Here's how the part is built. I have some questions about the finished solid (model axes, mm). Coordinates: 2 decimals unless noted, no trailing zeros. Loops run counter-clockwise (first coordinate to the right, second up) from the corner with the lowest first, then second, coordinate; pieces in that order, holes last. Notation, with made-up numbers: (31, 35.25) -> (67, 35.25) arc R32 cw to (67, 66.25) -> close; hole circle Ø7 at (-18.75, -4.5). An arc over 180 degrees is marked (long way). Answer as a JSON object with one key per item and string values. Group by question number.
Q1. I'm going to push flat-ended pins straight in: pin 1 (5 mm diameter, centred on x = -3.5, z = -1.5, fed in from -Y); pin 2 (5 mm diameter, centred on x = -7, z = -7.5, fed in from -Y). Where does each tip first touch, or does it pass through?
Q2. I want a section at C-C on z = 0.25. Write out the boundary of the cut face in (x, y), then the cut area to 3 significant figures.
Q3. I need wall thicknesses on line 1 (Z direction, x = -0.75, y = 0.05); line 2 (Z direction, x = 1.25, y = 0.8); line 3 (X direction, y = 0.25, z = -2). Which ranges of each line are inside material? Lowest first, please.
Q4. I want a section at A-A on y = 0. Write out the boundary of the cut face in (x, z), then the cut area to 3 significant figures.
Q5. I want a section at B-B on x = 4.5. Write out the boundary of the cut face in (y, z).
Autodesk Inventor part; units mm, degrees
ref_plane "YZ Plane" through (0, 0, 0) normal (1, 0, 0) x (0, 1, 0)
ref_plane "XZ Plane" through (0, 0, 0) normal (0, 1, 0) x (-1, 0, 0)
ref_plane "XY Plane" through (0, 0, 0) normal (0, 0, 1) x (1, 0, 0)
sketch "Эскиз1" plane through (0, 0, 0) normal (0, 1, 0) x (-1, 0, 0)
  line L0 (4.3898, 6.6229) -> (-5.6102, 6.6229)
  line L1 (-9.6102, 2.6229) -> (-9.6102, -7.3771)
  line L2 (-5.6102, -11.3771) -> (4.3898, -11.3771)
  line L3 (8.3898, -7.3771) -> (8.3898, 2.6229)
  arc A0 (8.3898, 2.6229) -> (4.3898, 6.6229) centre (4.3898, 2.6229) ccw
  arc A1 (4.3898, -11.3771) -> (8.3898, -7.3771) centre (4.3898, -7.3771) ccw
  arc A2 (-9.6102, -7.3771) -> (-5.6102, -11.3771) centre (-5.6102, -7.3771) ccw
  arc A3 (-5.6102, 6.6229) -> (-9.6102, 2.6229) centre (-5.6102, 2.6229) ccw
  point P0 (0, 0)
  point P1 (-9.6102, -11.3771)
  point P2 (-9.6102, 6.6229)
  point P3 (8.3898, -11.3771)
  point P4 (0, -11.3771)
  dimension "d0" = 18
  dimension "d1" = 18
  dimension "d2" = 4
sketch "Эскиз2" plane through (0, 0, 0) normal (0, 1, 0) x (-1, 0, 0)
  point P0 (0, 0)
ref_plane "РабПлоскость1" through (0, 0, -11.3771) normal (-1, 0, 0) x (0, -1, 0)
sketch "Эскиз3" plane through (0, 0, -11.3771) normal (-1, 0, 0) x (0, -1, 0)
  circle A0 centre (0, 0) radius 1.0246
  point P0 (0, 11.3771)
sweep "Сдвиг1" add profiles "Эскиз3" path "Эскиз1"
properties part number "Деталь 8 лаба"
Result set:
{
 "1": {"pin 1": "passes through", "pin 2": "stops at y = -1.02"},
 "2": {"outline": "circle Ø2.05 at (-8.39, 0); circle Ø2.05 at (9.61, 0)", "area": "6.60 mm²"},
 "3": {"line 1": "z = -12.4 to -10.35, 5.6 to 7.65", "line 2": "z = -12.02 to -10.74, 5.98 to 7.26", "line 3": "x = -9.38 to -7.4, 8.62 to 10.6"},
 "4": {"outline": "(-9.41, -7.38) arc R5.02 ccw to (-4.39, -12.4) -> (5.61, -12.4) arc R5.02 ccw to (10.63, -7.38) -> (10.63, 2.62) arc R5.02 ccw to (5.61, 7.65) -> (-4.39, 7.65) arc R5.02 ccw to (-9.41, 2.62) -> close; hole (-7.37, -7.38) arc R2.98 ccw to (-4.39, -10.35) -> (5.61, -10.35) arc R2.98 ccw to (8.59, -7.38) -> (8.59, 2.62) arc R2.98 ccw to (5.61, 5.6) -> (-4.39, 5.6) arc R2.98 ccw to (-7.37, 2.62) -> close", "area": "133 mm²"},
 "5": {"outline": "circle Ø2.05 at (0, -11.38); circle Ø2.05 at (0, 6.62)"}
}
